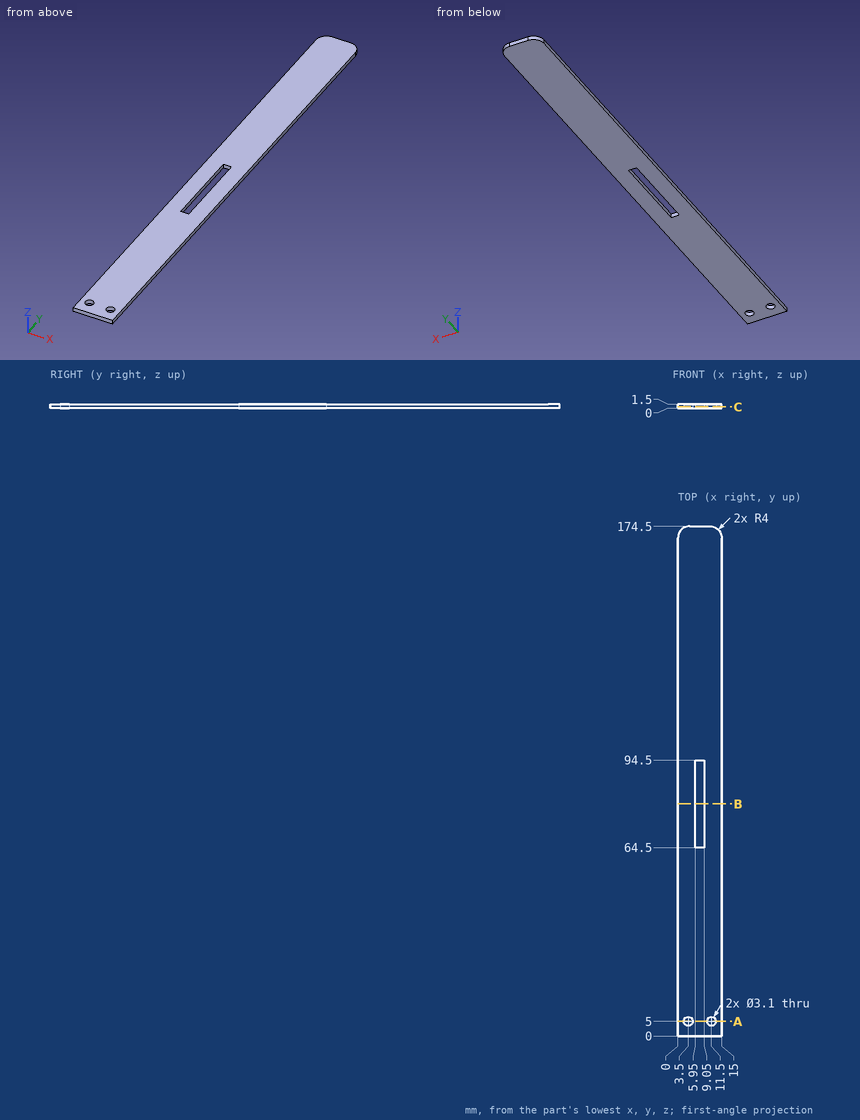
Could you check a few things on this drawing? It's one solid part, dimensions in mm from its lowest x, y, z. Give positions to 0.01 mm unless a question says otherwise; leave off trailing zeros. Loops run counter-clockwise (first coordinate to the right, second up) from the corner with the lowest first, then second, coordinate; pieces in that order, holes last. Notation, with made-up numbers: (87, -31.75) -> (104, -31.75) arc R8 cw to (104, -19.75) -> close; hole circle Ø5 at (10.25, 79). An arc over 180 degrees is marked (long way). Use one line per item in the form item = value. Start each with the question number.
1) Imagine slicing it at B-B (y = 79.5). Please give me the cut outline in (x, z).
2) For P1, Ø1.9, axis at x = 3.5, y = 5, coming from the +Z side, with a flat end and sliding along its axis, tell me the tip position at first contact or that it passes through.
3) Imagine slicing it at C-C (z = 0.55). Please give me the cut outline in (x, y).
4) Imagine slicing it at A-A (y = 5). Please give me the cut outline in (x, z).
5) Please list where these lines run through material, in increasing order: line 1 along X through (y, z) = (5, 1.15); line 2 along Y through (x, z) = (11.5, 0.4); line 3 along Y through (x, z) = (6.75, 0.7).
Check values:
q1.outline = (0, 0) -> (5.95, 0) -> (5.95, 1.5) -> (0, 1.5) -> close; (9.05, 0) -> (15, 0) -> (15, 1.5) -> (9.05, 1.5) -> close
q2.P1 = through
q3.outline = (0, 0) -> (15, 0) -> (15, 170.5) arc R4 ccw to (11, 174.5) -> (4, 174.5) arc R4 ccw to (0, 170.5) -> close; hole circle Ø3.1 at (3.5, 5); hole (5.95, 64.5) -> (9.05, 64.5) -> (9.05, 94.5) -> (5.95, 94.5) -> close; hole circle Ø3.1 at (11.5, 5)
q4.outline = (0, 0) -> (1.95, 0) -> (1.95, 1.5) -> (0, 1.5) -> close; (5.05, 0) -> (9.95, 0) -> (9.95, 1.5) -> (5.05, 1.5) -> close; (13.05, 0) -> (15, 0) -> (15, 1.5) -> (13.05, 1.5) -> close
q5.line_1 = 0 to 1.95, 5.05 to 9.95, 13.05 to 15
q5.line_2 = 0 to 3.45, 6.55 to 174.47
q5.line_3 = 0 to 64.5, 94.5 to 174.5
